Source: CAD feature listing. Evaluate the final solid. Frame: model axes, mm. Face numbers are marked on the shaded views. A direction names the side the tool comes from. Coordinates: 2 decimals unless noted, no trailing zeros. Write each loop counter-clockwise with the first axis right and the second up, starting at its lowest first coordinate (ties: lowest second). Pieces come first, ordered by that corner, then holes. Notation, with made-up numbers: (-31, 9.25) - (-22, 9.25) arc R35 cw to (-22, 48.25) - close; hole circle Ø9 at (42, -32.75). An arc over 180 degrees is marked (long way). One line per item, written item: value.
from build123d import *

# Parameters (mm, degrees)
BOSS_EXTRUDE1_DEPTH     = 30
CUT_EXTRUDE1_START      = 4
CUT_EXTRUDE1_DEPTH      = 30
SKETCH3_R               = 2
CUT_EXTRUDE2_DEPTH      = 9.5
CUT_EXTRUDE3_START      = 15
CUT_EXTRUDE3_DEPTH      = 20
CUT_EXTRUDE4_DEPTH      = 20
CUT_EXTRUDE4_DEPTH_BACK = 20
SKETCH5_R               = 7.5


with BuildPart() as part:
    # Sketch1 → Boss-Extrude1 (new body)
    with BuildSketch(Plane(origin=(0, 0, 0), x_dir=(1, 0, 0), z_dir=(0, 1, 0))):
        with BuildLine():
            Line((9.013878189, 15), (75, 15))
            Line((75, 15), (75, 5.549099401))
            Line((75, 5.549099401), (16.596912238, 5.549099401))
            ThreePointArc((16.596912238, 5.549099401), (17.493415402, -0.480018296), (16.26763294, -6.450900599))
            Line((16.26763294, -6.450900599), (75, -6.450900599))
            Line((75, -6.450900599), (75, -15))
            Line((75, -15), (9.013878189, -15))
            ThreePointArc((9.013878189, -15), (-17.5, 0), (9.013878189, 15))
        make_face()
    extrude(amount=BOSS_EXTRUDE1_DEPTH)

    # Sketch2 → Cut-Extrude1 (cut)
    with BuildSketch(Plane(origin=(0, 0, 0), x_dir=(1, 0, 0), z_dir=(0, 1, 0)).offset(CUT_EXTRUDE1_START)):
        with BuildLine():
            Line((8.75, 15.155444566), (7.5, 12.990381057))
            ThreePointArc((7.5, 12.990381057), (0, -15), (-7.5, 12.990381057))
            Line((-7.5, 12.990381057), (-8.75, 15.155444566))
            ThreePointArc((-8.75, 15.155444566), (-4.529333289, 16.90370196), (0, 17.5))
            ThreePointArc((0, 17.5), (4.529333289, 16.90370196), (8.75, 15.155444566))
        make_face()
    extrude(amount=CUT_EXTRUDE1_DEPTH, mode=Mode.SUBTRACT)

    # Sketch3 → Cut-Extrude2 (cut)
    with BuildSketch(Plane(origin=(0, 0, 0), x_dir=(1, 0, 0), z_dir=(0, 1, 0))):
        with Locations(Location((6.717514421, 6.717514421, 0), (0, 0, 270))):
            Circle(SKETCH3_R)
        with Locations(Location((6.717514421, -6.717514421, 0), (0, 0, 270))):
            Circle(SKETCH3_R)
        with Locations(Location((-6.717514421, -6.717514421, 0), (0, 0, 270))):
            Circle(SKETCH3_R)
        with Locations(Location((-6.717514421, 6.717514421, 0), (0, 0, 270))):
            Circle(SKETCH3_R)
    extrude(amount=CUT_EXTRUDE2_DEPTH, mode=Mode.SUBTRACT)

    # Sketch4 → Cut-Extrude3 (cut)
    with BuildSketch(Plane(origin=(0, 0, 0), x_dir=(1, 0, 0), z_dir=(0, 1, 0)).offset(CUT_EXTRUDE3_START)):
        with BuildLine():
            Line((8.75, -15.155444566), (0, 0))
            Line((0, 0), (8.75, 15.155444566))
            ThreePointArc((8.75, 15.155444566), (-17.5, 0), (8.75, -15.155444566))
        make_face()
    extrude(amount=CUT_EXTRUDE3_DEPTH, mode=Mode.SUBTRACT)

    # Sketch5 → Cut-Extrude4 (cut, two sides: drawn at the far end of the back side and taken through both)
    with BuildSketch(Plane.XY.offset(-CUT_EXTRUDE4_DEPTH_BACK)):
        with Locations(Location((62.5, 15, 0), (0, 0, 180))):
            Circle(SKETCH5_R)
        with Locations(Location((37.5, 15, 0), (0, 0, 180))):
            Circle(SKETCH5_R)
    extrude(amount=CUT_EXTRUDE4_DEPTH + CUT_EXTRUDE4_DEPTH_BACK, mode=Mode.SUBTRACT)


solid = part.part
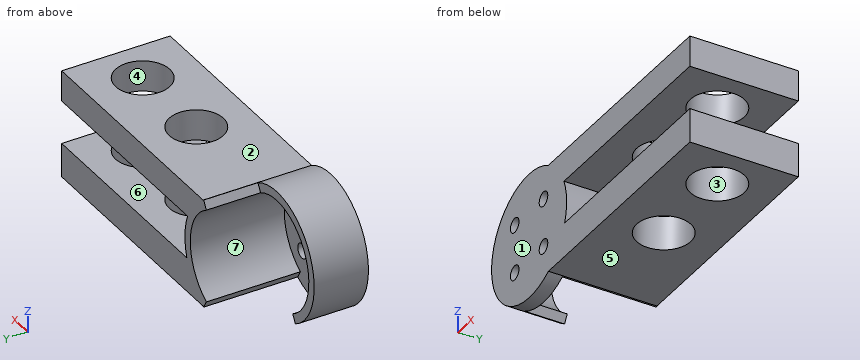
1) Draft query along Y for the marked faces 1, 2, 3 and 4. Return one class per face: released by +Y, released by -Y, zero draft, split by the parting line, or undercut.
Values found:
face 1: released by -Y
face 2: zero draft
face 3: undercut
face 4: undercut
2) Material intervals for line 1 (Z direction, x = 49, y = 21); line 2 (Y direction, x = 37.5, z = -7.75); line 3 (X direction, y = 16.5, z = -8.5), sorted ascending.
Values found:
line 1: -15 to -5.55, 6.45 to 15
line 2: 0 to 7.5, 22.5 to 30
line 3: 12.36 to 30.15, 44.85 to 55.15, 69.85 to 75
3) Reachability of the marked faces 5, 6 and 7 from +Z, -Z, +X, -X, +Y, -Y: full face, straight path, thin tool, end or side. Return the list, or none.
Values found:
face 5: -Z, +X, +Y, -Y
face 6: +X, +Y, -Y
face 7: +Y
4) Section query A-A on x = 62.5. Output: boundary loops of the cut face in (y, z).
Values found:
outline: (0, -15) - (7.5, -15) - (7.5, -5.55) - (0, -5.55) - close; (0, 6.45) - (7.5, 6.45) - (7.5, 15) - (0, 15) - close; (22.5, -15) - (30, -15) - (30, -5.55) - (22.5, -5.55) - close; (22.5, 6.45) - (30, 6.45) - (30, 15) - (22.5, 15) - close
5) Section query D-D on z = 0. Output: boundary loops of the cut face in (x, y), then the cut area to 4 significant figures.
Values found:
outline: (-17.5, 0) - (17.5, 0) - (17.5, 30) - (15, 30) - (15, 4) - (-15, 4) - (-15, 15) - (-17.5, 15) - close
area: 232.5 mm2
6) Section query B-B on x = 24.5. Output: boundary loops of the cut face in (y, z).
Values found:
outline: (0, -15) - (30, -15) - (30, -5.55) - (0, -5.55) - close; (0, 6.45) - (30, 6.45) - (30, 15) - (0, 15) - close
7) Contact query for flat-ended pins moving along their axis: P1, Ø2, axis at y = 12.5, z = 1.5, coming from the -X side; P2, Ø21, axis at x = -10, z = -5.5, coming from the +Y side; P3, Ø5, axis at x = 8, z = 1, coming from the +Y side. Output: stop coordinate, or through.
Values found:
P1: x = -17.49
P2: y = 15
P3: y = 4
8) Section query C-C on y = 11. Output: boundary loops of the cut face in (x, z).
Values found:
outline: (-8.75, -15.16) - (-7.5, -12.99) arc R15 cw (long way) to (7.5, -12.99) - (8.75, -15.16) arc R17.5 ccw to (9.01, -15) - (31.16, -15) - (31.16, -5.55) - (16.6, -5.55) arc R17.5 ccw to (16.27, 6.45) - (31.16, 6.45) - (31.16, 15) - (9.01, 15) arc R17.5 ccw (long way) to start; (43.84, -15) - (56.16, -15) - (56.16, -5.55) - (43.84, -5.55) - close; (43.84, 6.45) - (56.16, 6.45) - (56.16, 15) - (43.84, 15) - close; (68.84, -15) - (75, -15) - (75, -5.55) - (68.84, -5.55) - close; (68.84, 6.45) - (75, 6.45) - (75, 15) - (68.84, 15) - close
